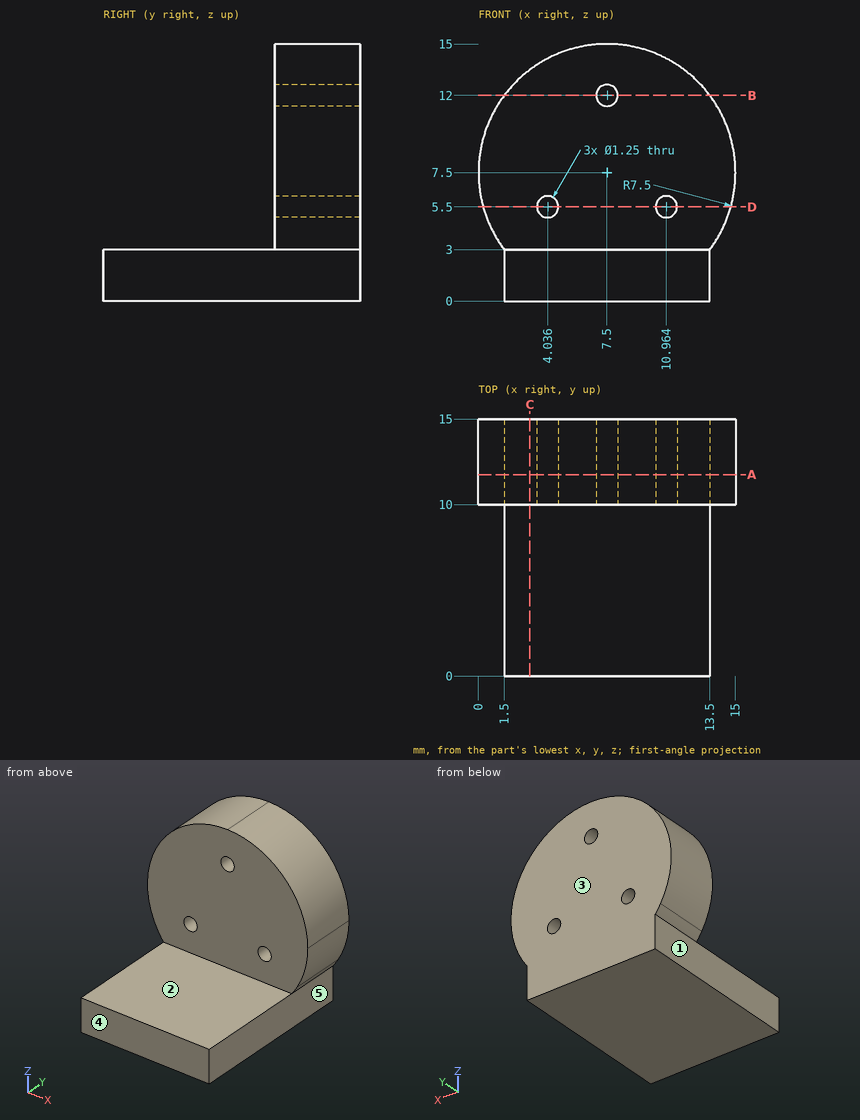
Verification items for this drawing (mm, ordinates from the low corner). A direction names the side the tool comes from. Coordinates: 2 decimals unless noted, no trailing zeros. Loops run counter-clockwise (first coordinate to the right, second up) from the corner with the lowest first, then second, coordinate; pieces in that order, holes last. Notation, with made-up numbers: (87.5, 75.5) - (91.5, 75.5) arc R19 cw to (91.5, 108.5) - close; hole circle Ø5 at (47, 69). An arc over 180 degrees is marked (long way). Use one line per item in the form item = value. Start each with the question number.
Item 1: Section check B-B, the plane z = 12. Enter the section's corners in (x, y) (3 decimals).
Item 2: Gauge pin test, flat ends, axial feed: pin 1 (6 mm diameter, centred on x = 2, y = 13.5, fed in from +Z); pin 2 (5 mm diameter, centred on x = 5, z = 4, fed in from -Y); pin 3 (3.5 mm diameter, centred on x = 7, z = 9, fed in from -Y); pin 4 (3 mm diameter, centred on x = 5.5, y = 6.5, fed in from +Z). Record the tip position at first contact, or that the pin passes through.
Item 3: Section check D-D, the plane z = 5.5. Enter the section's corners in (x, y), and give its area (3 significant figures).
Item 4: Tool access check on the marked faces 1, 2, 3, 4 and 5. Record the directions out of +Z, -Z, +X, -X, +Y, -Y that give a thin tool (end or side, any length) a straight path to the whole face; none if there is none.
Item 5: Section check C-C, the plane x = 3. Enter the section's corners in (y, z), and give its area (3 significant figures).
Item 6: Section check A-A, the plane y = 11.75. Enter the section's corners in (x, z) (3 decimals), and give its area (3 significant figures).
Item 7: Thickness scan on probe 1 along X at (y, z) = (13.2, 5.5); probe 2 along Z at (x, y) = (12.5, 1.75); probe 3 along Y at (x, z) = (12, 4.25). Record the ranges inside material, lowest first.
Computed:
q1.outline = (1.5, 10) - (6.875, 10) - (6.875, 15) - (1.5, 15) - close; (8.125, 10) - (13.5, 10) - (13.5, 15) - (8.125, 15) - close
q2.pin_1 = 14.57
q2.pin_2 = 0
q2.pin_3 = 10
q2.pin_4 = 3
q3.outline = (0.27, 10) - (3.41, 10) - (3.41, 15) - (0.27, 15) - close; (4.66, 10) - (10.34, 10) - (10.34, 15) - (4.66, 15) - close; (11.59, 10) - (14.73, 10) - (14.73, 15) - (11.59, 15) - close
q3.area = 59.8 mm2
q4.face_1 = -Z, -X, +Y, -Y
q4.face_2 = +Z, +X, -X, -Y
q4.face_3 = +Z, -Z, +X, -X, +Y
q4.face_4 = +Z, -Z, +X, -X, -Y
q4.face_5 = -Z, +X, +Y, -Y
q5.outline = (0, 0) - (15, 0) - (15, 13.5) - (10, 13.5) - (10, 3) - (0, 3) - close
q5.area = 97.5 mm2
q6.outline = (1.5, 0) - (13.5, 0) - (13.5, 3) arc R7.5 ccw (long way) to (1.5, 3) - close; hole circle Ø1.25 at (4.036, 5.5); hole circle Ø1.25 at (7.5, 12); hole circle Ø1.25 at (10.964, 5.5)
q6.area = 184 mm2
q7.probe_1 = 0.27 to 3.41, 4.66 to 10.34, 11.59 to 14.73
q7.probe_2 = 0 to 3
q7.probe_3 = 10 to 15
